from build123d import *

# Parameters (mm, degrees)
SKETCH1_R           = 5
BOSS_EXTRUDE1_DEPTH = 10
SKETCH2_R           = 5
BOSS_EXTRUDE2_DEPTH = 10


with BuildPart() as part:
    # Sketch1 → Boss-Extrude1 (new body, symmetric)
    with BuildSketch(Plane.XY):
        Circle(SKETCH1_R)
    extrude(amount=BOSS_EXTRUDE1_DEPTH, both=True)

    # Sketch2 → Boss-Extrude2 (add, symmetric)
    with BuildSketch(Plane(origin=(0, 0, 0), x_dir=(1, 0, 0), z_dir=(0, 1, 0))):
        Circle(SKETCH2_R)
    extrude(amount=BOSS_EXTRUDE2_DEPTH, both=True)


solid = part.part
The model under review builds one solid part; all positions refer to its coordinate system, in mm. A direction names the side the tool comes from. Coordinates: 2 decimals unless noted, no trailing zeros. Loops run counter-clockwise (first coordinate to the right, second up) from the corner with the lowest first, then second, coordinate; pieces in that order, holes last.
(1) Consider section C-C, the plane y = 3.5. Give the boundary of the cut face in (x, z).
Determined:
outline: (-3.57, -10) - (3.57, -10) - (3.57, -3.5) arc R5 ccw to (3.57, 3.5) - (3.57, 10) - (-3.57, 10) - (-3.57, 3.5) arc R5 ccw to (-3.57, -3.5) - close
(2) Consider section A-A, the plane x = 0. Give the boundary of the cut face in (y, z).
Determined:
outline: (-10, -5) - (-5, -5) - (-5, -10) - (5, -10) - (5, -5) - (10, -5) - (10, 5) - (5, 5) - (5, 10) - (-5, 10) - (-5, 5) - (-10, 5) - close
(3) Consider section B-B, the plane z = 8.75. Give the boundary of the cut face in (x, y), plus the area to 3 significant figures.
Determined:
outline: circle Ø10 at (0, 0)
area: 78.5 mm2
(4) Tool access review of faces 1 (the cylindrical face through (-4, 6, -3)), 2 (the cylindrical face through (-4, -6, 3)), 3 (the cylindrical face through (-4, 3, 6)): name each direction out of +Z, -Z, +X, -X, +Y, -Y from which nothing blocks a thin tool from reaching the whole face with its end or side.
Determined:
face 1: +Y
face 2: -Y
face 3: +Z
(5) Wall thickness on L1, parallel to Z at x = 2.75, y = -4.75; L2, parallel to X at y = -0.5, z = 1; L3, parallel to X at y = 2, z = -0.75: over which ranges is each line inside the solid? List them lowest first.
Determined:
L1: z = -4.18 to 4.18
L2: x = -4.97 to 4.97
L3: x = -4.94 to 4.94
(6) Insertion check: P1, Ø2, axis at y = 3, z = 6, coming from the +X side; P2, Ø3, axis at y = 4.5, z = 5, coming from the +X side; P3, Ø4, axis at x = 2, y = -7, coming from the +Z side. Each pin has a flat end and moves straight along its axis. Give the tip position at first contact, or say it passes through.
Determined:
P1: stops at x = 4.58
P2: stops at x = 4
P3: stops at z = 5
(7) Consider section D-D, the plane x = 2.5. Give the boundary of the cut face in (y, z).
Determined:
outline: (-10, -4.33) - (-4.33, -4.33) - (-4.33, -10) - (4.33, -10) - (4.33, -4.33) - (10, -4.33) - (10, 4.33) - (4.33, 4.33) - (4.33, 10) - (-4.33, 10) - (-4.33, 4.33) - (-10, 4.33) - close
